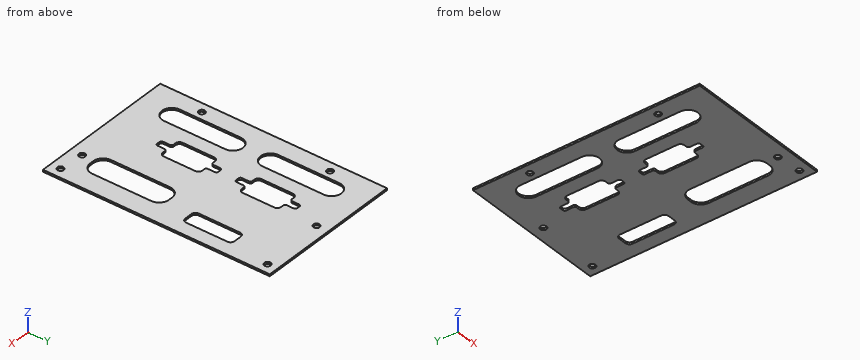
Autodesk Inventor part; units mm, degrees
ref_plane "YZ Plane" through (0, 0, 0) normal (1, 0, 0) x (0, 1, 0)
ref_plane "XZ Plane" through (0, 0, 0) normal (0, 1, 0) x (-1, 0, 0)
ref_plane "XY Plane" through (0, 0, 0) normal (0, 0, 1) x (1, 0, 0)
sketch "Sketch1" plane through (0, 0, 0) normal (0, 0, 1) x (1, 0, 0)
  line L0 (-37.5, 57.5) -> (37.5, 57.5)
  line L1 (37.5, 57.5) -> (37.5, -57.5)
  line L2 (37.5, -57.5) -> (-37.5, -57.5)
  line L3 (-37.5, -57.5) -> (-37.5, 57.5)
  line L4 (-37.5, 57.5) -> (37.5, -57.5) construction
  line L5 (37.5, 57.5) -> (-37.5, -57.5) construction
  line L6 (0, 0) -> (0, 12.9993)
  circle A0 centre (-32.6, -32.5) radius 1.6
  circle A1 centre (0, 51.5) radius 1.6
  line L7 (0, 0) -> (8.7382, 0)
  circle A2 centre (20, -51.5) radius 1.6
  circle A3 centre (-32.6, 32.5) radius 1.6
  circle A4 centre (32.6, 52.5) radius 1.6
  circle A5 centre (32.6, -52.5) radius 1.6
  line L8 (0.6, -9.5) -> (0.6, -25.5)
  line L9 (-11.4, -25.5) -> (-11.4, -9.5)
  line L10 (-11.4, -7.5) -> (0.6, -27.5) construction
  line L11 (0.6, -7.5) -> (-11.4, -27.5) construction
  line L12 (-6.15, -2) -> (-4.65, -2)
  line L13 (-3.65, -3) -> (-3.65, -6.5)
  line L14 (-7.15, -6.5) -> (-7.15, -3)
  line L15 (-7.15, -2) -> (-3.65, -7.5) construction
  line L16 (-3.65, -2) -> (-7.15, -7.5) construction
  line L17 (-6.15, -33) -> (-4.65, -33)
  line L18 (-3.65, -32) -> (-3.65, -28.5)
  line L19 (-7.15, -28.5) -> (-7.15, -32)
  line L20 (-7.15, -33) -> (-3.65, -27.5) construction
  line L21 (-3.65, -33) -> (-7.15, -27.5) construction
  line L22 (28.5, 7.5) -> (24.5, 7.5)
  line L23 (22.5, 9.5) -> (22.5, 30.5)
  line L24 (24.5, 32.5) -> (28.5, 32.5)
  line L25 (30.5, 30.5) -> (30.5, 9.5)
  line L26 (30.5, 7.5) -> (22.5, 32.5) construction
  line L27 (22.5, 7.5) -> (30.5, 32.5) construction
  line L28 (-23.5, -45.5) -> (-23.5, -45.5)
  line L29 (-28.5, -40.5) -> (-28.5, -9.5)
  line L30 (-23.5, -4.5) -> (-23.5, -4.5)
  line L31 (-18.5, -9.5) -> (-18.5, -40.5)
  line L32 (-18.5, -45.5) -> (-28.5, -4.5) construction
  line L33 (-28.5, -45.5) -> (-18.5, -4.5) construction
  arc A6 (-23.5, -45.5) -> (-18.5, -40.5) centre (-23.5, -40.5) ccw
  arc A7 (-18.5, -9.5) -> (-23.5, -4.5) centre (-23.5, -9.5) ccw
  arc A8 (-23.5, -4.5) -> (-28.5, -9.5) centre (-23.5, -9.5) ccw
  arc A9 (-28.5, -40.5) -> (-23.5, -45.5) centre (-23.5, -40.5) ccw
  line L34 (-23.5, 45.5) -> (-23.5, 45.5)
  line L35 (-28.5, 40.5) -> (-28.5, 9.5)
  line L36 (-23.5, 4.5) -> (-23.5, 4.5)
  line L37 (-18.5, 9.5) -> (-18.5, 40.5)
  line L38 (-18.5, 45.5) -> (-28.5, 4.5) construction
  line L39 (-28.5, 45.5) -> (-18.5, 4.5) construction
  arc A10 (-18.5, 40.5) -> (-23.5, 45.5) centre (-23.5, 40.5) ccw
  arc A11 (-23.5, 4.5) -> (-18.5, 9.5) centre (-23.5, 9.5) ccw
  arc A12 (-28.5, 9.5) -> (-23.5, 4.5) centre (-23.5, 9.5) ccw
  arc A13 (-23.5, 45.5) -> (-28.5, 40.5) centre (-23.5, 40.5) ccw
  line L40 (22.5, -45.5) -> (20.5, -45.5)
  line L41 (15.5, -40.5) -> (15.5, -10.5)
  line L42 (20.5, -5.5) -> (22.5, -5.5)
  line L43 (27.5, -10.5) -> (27.5, -40.5)
  line L44 (27.5, -45.5) -> (15.5, -5.5) construction
  line L45 (15.5, -45.5) -> (27.5, -5.5) construction
  arc A14 (22.5, -45.5) -> (27.5, -40.5) centre (22.5, -40.5) ccw
  arc A15 (15.5, -40.5) -> (20.5, -45.5) centre (20.5, -40.5) ccw
  arc A16 (27.5, -10.5) -> (22.5, -5.5) centre (22.5, -10.5) ccw
  arc A17 (20.5, -5.5) -> (15.5, -10.5) centre (20.5, -10.5) ccw
  arc A18 (-7.15, -32) -> (-6.15, -33) centre (-6.15, -32) ccw
  arc A19 (-4.65, -33) -> (-3.65, -32) centre (-4.65, -32) ccw
  arc A20 (-3.65, -3) -> (-4.65, -2) centre (-4.65, -3) ccw
  arc A21 (-6.15, -2) -> (-7.15, -3) centre (-6.15, -3) ccw
  line L46 (-9.4, -7.5) -> (-8.15, -7.5)
  line L47 (-2.65, -7.5) -> (-1.4, -7.5)
  line L48 (-1.4, -27.5) -> (-2.65, -27.5)
  line L49 (-8.15, -27.5) -> (-9.4, -27.5)
  arc A22 (-1.4, -27.5) -> (0.6, -25.5) centre (-1.4, -25.5) ccw
  arc A23 (0.6, -9.5) -> (-1.4, -7.5) centre (-1.4, -9.5) ccw
  arc A24 (-11.4, -25.5) -> (-9.4, -27.5) centre (-9.4, -25.5) ccw
  arc A25 (-9.4, -7.5) -> (-11.4, -9.5) centre (-9.4, -9.5) ccw
  arc A26 (-7.15, -28.5) -> (-8.15, -27.5) centre (-8.15, -28.5) ccw
  arc A27 (-2.65, -27.5) -> (-3.65, -28.5) centre (-2.65, -28.5) ccw
  arc A28 (-3.65, -6.5) -> (-2.65, -7.5) centre (-2.65, -6.5) ccw
  arc A29 (-8.15, -7.5) -> (-7.15, -6.5) centre (-8.15, -6.5) ccw
  line L50 (-7.15, 11.5) -> (-7.15, 8)
  arc A30 (-2.65, 12.5) -> (-3.65, 11.5) centre (-2.65, 11.5) ccw
  arc A31 (-1.4, 12.5) -> (0.6, 14.5) centre (-1.4, 14.5) ccw
  line L51 (-1.4, 12.5) -> (-2.65, 12.5)
  arc A32 (-7.15, 8) -> (-6.15, 7) centre (-6.15, 8) ccw
  line L52 (-7.15, 7) -> (-3.65, 12.5) construction
  line L53 (-3.65, 7) -> (-7.15, 12.5) construction
  line L54 (-3.65, 8) -> (-3.65, 11.5)
  line L55 (-6.15, 7) -> (-4.65, 7)
  arc A33 (-4.65, 7) -> (-3.65, 8) centre (-4.65, 8) ccw
  line L56 (-11.4, 14.5) -> (-11.4, 30.5)
  arc A34 (-7.15, 11.5) -> (-8.15, 12.5) centre (-8.15, 11.5) ccw
  line L57 (-8.15, 12.5) -> (-9.4, 12.5)
  arc A35 (-11.4, 14.5) -> (-9.4, 12.5) centre (-9.4, 14.5) ccw
  line L58 (-2.65, 32.5) -> (-1.4, 32.5)
  arc A36 (0.6, 30.5) -> (-1.4, 32.5) centre (-1.4, 30.5) ccw
  line L59 (-6.15, 38) -> (-4.65, 38)
  line L60 (-3.65, 37) -> (-3.65, 33.5)
  line L61 (-7.15, 33.5) -> (-7.15, 37)
  line L62 (-7.15, 38) -> (-3.65, 32.5) construction
  line L63 (-3.65, 38) -> (-7.15, 32.5) construction
  line L64 (-9.4, 32.5) -> (-8.15, 32.5)
  arc A37 (-8.15, 32.5) -> (-7.15, 33.5) centre (-8.15, 33.5) ccw
  arc A38 (-9.4, 32.5) -> (-11.4, 30.5) centre (-9.4, 30.5) ccw
  arc A39 (-6.15, 38) -> (-7.15, 37) centre (-6.15, 37) ccw
  arc A40 (-3.65, 37) -> (-4.65, 38) centre (-4.65, 37) ccw
  arc A41 (-3.65, 33.5) -> (-2.65, 32.5) centre (-2.65, 33.5) ccw
  line L65 (0.6, 30.5) -> (0.6, 14.5)
  line L66 (-11.4, 32.5) -> (0.6, 12.5) construction
  line L67 (0.6, 32.5) -> (-11.4, 12.5) construction
  arc A42 (24.5, 32.5) -> (22.5, 30.5) centre (24.5, 30.5) ccw
  arc A43 (30.5, 30.5) -> (28.5, 32.5) centre (28.5, 30.5) ccw
  arc A44 (28.5, 7.5) -> (30.5, 9.5) centre (28.5, 9.5) ccw
  arc A45 (22.5, 9.5) -> (24.5, 7.5) centre (24.5, 9.5) ccw
  point P0 (-5.4, -17.5)
  point P1 (-5.4, -4.75)
  point P2 (-5.4, -30.25)
  point P3 (26.5, 20)
  point P4 (-23.5, -25)
  point P5 (-23.5, 25)
  point P6 (21.5, -25.5)
  point P7 (-5.4, 9.75)
  point P8 (-5.4, 35.25)
  point P9 (-5.4, 22.5)
  point P10 (0, 57.5)
  point P11 (0, -57.5)
  point P12 (22.5, 20)
  dimension "d0" = 115
  dimension "d1" = 75
  dimension "d22" = 3.2
  dimension "d25" = 3.2
  dimension "d26" = 6
  dimension "d27" = 25
  dimension "d28" = 4.9
  dimension "d29" = 3.2
  dimension "d30" = 4.9
  dimension "d31" = 5
  dimension "d32" = 5.5
  dimension "d33" = 3.5
  dimension "d34" = 12
  dimension "d35" = 20
  dimension "d38" = 26.1
  dimension "d39" = 8
  dimension "d40" = 25
  dimension "d42" = 25
  dimension "d43" = 41
  dimension "d44" = 10
  dimension "d45" = 9
  dimension "d46" = 12
  dimension "d47" = 5
  dimension "d48" = 40
  dimension "d49" = 12
  dimension "d50" = 10
  dimension "d51" = 12
  dimension "d52" = 5
  dimension "d53" = 1
  dimension "d54" = 30
  dimension "d55" = 2
  dimension "d56" = 1
  dimension "d59" = 40
  dimension "d64" = 9
  dimension "d65" = 12
  dimension "d67" = 0
  dimension "d68" = 3.2
  dimension "d69" = 6
  dimension "d70" = 20
  dimension "d71" = 2
  dimension "d72" = 60
extrude "Plate1" add sketch "Sketch1" along normal blind 1
equation "\"d2\" = 厚度"
equation "\"折彎半徑\" = 厚度"
equation "\"折彎離隙寬度\" = 厚度"
equation "\"折彎離隙深度\" = 0.5 * 厚度"
equation "\"轉角離隙大小\" = 4 * 厚度"
equation "\"最小剩餘\" = 2 * 厚度"
equation "\"轉移半徑\" = 折彎半徑"
equation "\"Jacobi半徑大小\" = 折彎半徑"
equation "\"間隙大小\" = 厚度"
properties part number "PCB_board_box_front" material "Aluminum"
Can you work these out from the model? Positions are in its coordinate system, mm. Give positions to 0.01 mm unless a question says otherwise; leave off trailing zeros. Write each loop counter-clockwise with the first axis right and the second up, starting at its lowest first coordinate (ties: lowest second). Pieces come first, ordered by that corner, then holes. Notation, with made-up numbers: M 28.5,-16 L 44.5,-16 A22 ccw 44.5,1 Z; hole C 30,12.5 d8. An arc over 180 degrees is marked long. Answer in a Markdown table with one row per item. Add a question column.
Item 1: Please list where these lines run through material, in increasing order: L1, parallel to Y at x = -32.6, z = 0.25; L2, parallel to X at y = -12.5, z = 0.85; L3, parallel to X at y = 16.5, z = 0.35.
Item 2: Imagine slicing it at A-A, the plane x = -22. Write out the boundary of the cut face in (y, z).
Item 3: Imagine slicing it at B-B, the plane z = 0.2. State how many separate pieces and enclosed holes the cut face has, plus the area to 3 significant figures.
Evaluation:
| question | item | result |
|---|---|---|
| 1 | L1 | y = -57.5 to -34.1, -30.9 to 30.9, 34.1 to 57.5 |
| 1 | L2 | x = -37.5 to -28.5, -18.5 to -11.4, 0.6 to 15.5, 27.5 to 37.5 |
| 1 | L3 | x = -37.5 to -28.5, -18.5 to -11.4, 0.6 to 22.5, 30.5 to 37.5 |
| 2 | outline | M -57.5,0 L -45.27,0 L -45.27,1 L -57.5,1 Z; M -4.73,0 L 4.73,0 L 4.73,1 L -4.73,1 Z; M 45.27,0 L 57.5,0 L 57.5,1 L 45.27,1 Z |
| 3 | separate pieces | 1 |
| 3 | enclosed holes | 12 |
| 3 | area | 6,590 mm² |
